```python
from build123d import *

# Parameters (mm, degrees)
SKETCH1_W           = 180
SKETCH1_H           = 360
BOSS_EXTRUDE1_DEPTH = 20
SKETCH2_R           = 30
SKETCH2_W           = 60
SKETCH2_H           = 30
SKETCH2_W_2         = 61.624654561
SKETCH2_H_2         = 60
CUT_EXTRUDE1_DEPTH  = 3


with BuildPart() as part:
    # Sketch1 → Boss-Extrude1 (new body)
    with BuildSketch(Plane(origin=(0, 0, 0), x_dir=(1, 0, 0), z_dir=(0, 1, 0))):
        Rectangle(SKETCH1_W, SKETCH1_H)
    extrude(amount=-BOSS_EXTRUDE1_DEPTH)

    # Sketch2 → Cut-Extrude1 (cut)
    with BuildSketch(Plane(origin=(0, 0, 0), x_dir=(1, 0, 0), z_dir=(0, 1, 0))):
        with Locations((34.656170811, 130)):
            Circle(SKETCH2_R)
        with Locations((34.656170811, -55.914468779)):
            Circle(SKETCH2_R)
        with Locations((-40, 47.162192329)):
            Rectangle(SKETCH2_W, SKETCH2_H)
        with Locations((-39.18767272, 130)):
            Rectangle(SKETCH2_W_2, SKETCH2_H_2)
        Polygon((4.656170811, 32.162192329), (64.656170811, 32.162192329), (34.656170811, 84.123716556), align=None)
        Polygon((4.656170811, -160.040110734), (64.656170811, -160.040110734), (34.656170811, -108.078586507), align=None)
        with Locations((-40, -142.801384824)):
            Rectangle(SKETCH2_W, SKETCH2_H)
        Polygon((-8.375345439, -25.441495932), (-8.375345439, -86.387441626), (-70, -86.387441626), (-70, -26.387441626), align=None)
    extrude(amount=-CUT_EXTRUDE1_DEPTH, mode=Mode.SUBTRACT)


solid = part.part
```
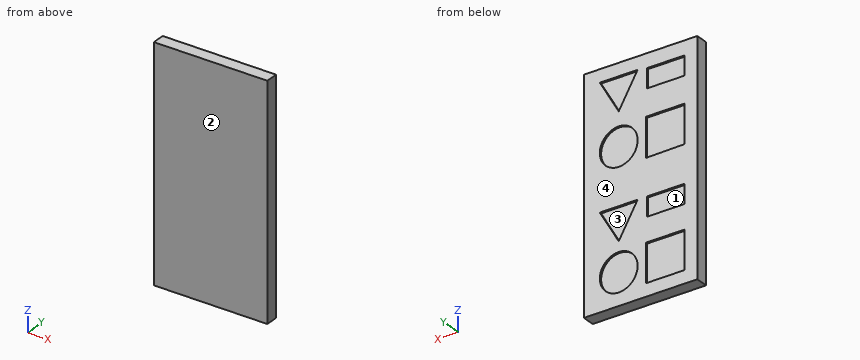
Geometry check sheet. Reference: the model listing, model coordinates, mm. Face numbers are marked on the shaded views. A direction names the side the tool comes from. Give positions to 0.01 mm unless a question says otherwise; leave off trailing zeros. Write each loop counter-clockwise with the first axis right and the second up, starting at its lowest first coordinate (ties: lowest second). Pieces come first, ordered by that corner, then holes. Notation, with made-up numbers: (65, -18) - (106, -18) arc R7 cw to (106, -13) - close; hole circle Ø11 at (-3, -20). An arc over 180 degrees is marked (long way). Use a Markdown table: item, result.
Q1. Section check C-C, the plane x = 18.5. Enter the section's corners in (y, z), then the cut area to 3 significant figures.
Computed:
| item | result |
|---|---|
| outline | (-20, -180) - (0, -180) - (0, -155.28) - (-3, -155.28) - (-3, -104.72) - (0, -104.72) - (0, -56.14) - (-3, -56.14) - (-3, -32.16) - (0, -32.16) - (0, 30.64) - (-3, 30.64) - (-3, 81.19) - (0, 81.19) - (0, 136.06) - (-3, 136.06) - (-3, 160.04) - (0, 160.04) - (0, 180) - (-20, 180) - close |
| area | 6,750 mm² |
Q2. Thickness scan on L1, parallel to X at y = -1.15, z = -130; L2, parallel to Y at x = 50, z = 158.5. Record the ranges inside material, lowest first. Write a range as [from, to].
Computed:
| item | result |
|---|---|
| L1 | x = [-90, -70], [-8.38, 4.66], [64.66, 90] |
| L2 | y = [-20, -3] |
Q3. Section check B-B, the plane x = -21. Enter the section's corners in (y, z).
Computed:
| item | result |
|---|---|
| outline | (-20, -180) - (0, -180) - (0, -160) - (-3, -160) - (-3, -100) - (0, -100) - (0, -62.16) - (-3, -62.16) - (-3, -32.16) - (0, -32.16) - (0, 25.64) - (-3, 25.64) - (-3, 86.39) - (0, 86.39) - (0, 127.8) - (-3, 127.8) - (-3, 157.8) - (0, 157.8) - (0, 180) - (-20, 180) - close |
Q4. Set-up check for the marked faces 3 and 4: record each of +Z, -Z, +X, -X, +Y, -Y from which the full face is reachable in a straight line by a thin tool's end or side.
Computed:
| item | result |
|---|---|
| face 3 | +Y |
| face 4 | +Z, -Z, +X, -X, +Y |
Q5. Go/stop test with a flat-tipped pin: P1, Ø1, axis at x = -40.5, z = 38, coming from the +Y side. Record where the tip stops, or that it passes through.
Computed:
| item | result |
|---|---|
| P1 | stops at y = -3 |
Q6. Section check A-A, the plane z = -130. Enter the section's corners in (x, y), then the cut area to 3 significant figures.
Computed:
| item | result |
|---|---|
| outline | (-90, -20) - (90, -20) - (90, 0) - (64.66, 0) - (64.66, -3) - (4.66, -3) - (4.66, 0) - (-8.38, 0) - (-8.38, -3) - (-70, -3) - (-70, 0) - (-90, 0) - close |
| area | 3,240 mm² |
Q7. Draft check along X on the marked faces 1 and 2. Enter one of: pulls with the +X half, pulls with the -X half, needs draft (parallel to the pull), parting line crosses it, or undercut.
Computed:
| item | result |
|---|---|
| face 1 | undercut |
| face 2 | needs draft |
